Autodesk Inventor part; units mm, degrees
ref_plane "Work Plane1" through (119.25, -2.5, 0) normal (1, 0, 0) x (0, 0, -1)
ref_plane "YZ Plane" through (0, 0, 0) normal (1, 0, 0) x (0, 1, 0)
ref_plane "XZ Plane" through (0, 0, 0) normal (0, 1, 0) x (-1, 0, 0)
sketch "Sketch2" plane through (0, 0, 0) normal (0, 0, 1) x (1, 0, 0)
  line L0 (-124.5, 2.5) -> (124.5, 2.5)
  line L1 (124.5, 2.5) -> (124.5, -2.5)
  line L2 (124.5, -2.5) -> (-124.5, -2.5)
  line L3 (-124.5, -2.5) -> (-124.5, 2.5)
  point P0 (0, 0)
  dimension "d1" = 249
  dimension "d2" = 5
  dimension "d3" = 2.5
  dimension "d4" = 124.5
sketch "Sketch3" plane through (0, 0, 0) normal (1, 0, 0) x (0, 1, 0)
  line L0 (0, 0) -> (-53.033, 53.033)
  line L1 (0, -0.5221) -> (1.6531, -0.5221)
  dimension "d5" = 75
  dimension "d6" = 45
sweep "Sweep1" add profiles "Sketch2" path "Sketch3" path curves L0
sketch "Sketch10" plane through (124.5, 2.5, 0) normal (0, 0, -1) x (-1, 0, 0)
  line L0 (249, 0) -> (0, 0)
  line L1 (0, 0) -> (0, -5)
  line L2 (0, -5) -> (249, -5)
  line L3 (249, -5) -> (249, 0)
  line L4 (15, 0) -> (234, 0)
  line L5 (234, 0) -> (234, -2)
  line L6 (234, -2) -> (15, -2)
  line L7 (15, -2) -> (15, 0)
  point P0 (124.5, -2.5)
  dimension "d76" = 2
  dimension "d77" = 219
  dimension "d78" = 109.5
extrude "Extrusion5" add sketch "Sketch10" along normal blind 10 contours L5 L6 L7 L0
sketch "Sketch11" plane through (-109.5, 0.5, 0) normal (0, -1, 0) x (1, 0, 0)
  line L0 (0, 0) -> (219, 0)
  line L1 (0, 0) -> (0, -10)
  line L2 (219, -10) -> (0, -10)
  line L3 (219, 0) -> (219, -10)
  line L4 (201.75, -6) -> (151.75, -6)
  line L5 (151.75, -6) -> (151.75, -4)
  line L6 (151.75, -4) -> (201.75, -4)
  line L7 (201.75, -4) -> (201.75, -6)
  line L8 (134.5, -6) -> (84.5, -6)
  line L9 (84.5, -6) -> (84.5, -4)
  line L10 (84.5, -4) -> (134.5, -4)
  line L11 (134.5, -4) -> (134.5, -6)
  line L12 (67.25, -6) -> (17.25, -6)
  line L13 (17.25, -6) -> (17.25, -4)
  line L14 (17.25, -4) -> (67.25, -4)
  line L15 (67.25, -4) -> (67.25, -6)
  point P0 (109.5, 0)
  dimension "d81" = 50
  dimension "d82" = 2
  dimension "d83" = 10
  dimension "d84" = 219
  dimension "d85" = 4
  dimension "d86" = 50
  dimension "d87" = 50
  dimension "d88" = 17.25
  dimension "d89" = 17.25
  dimension "d90" = 17.25
  dimension "d91" = 17.25
extrude "Extrusion6" add sketch "Sketch11" along normal blind 6 contours L4 L5 L6 L7 | L8 L9 L10 L11 | L12 L13 L14 L15
sketch "Sketch13" plane through (124.5, -2.5, 0) normal (1, 0, 0) x (0, 0, -1)
  line L0 (0, 5) -> (0, 0)
  line L1 (0, 5) -> (-53.033, -48.033)
  line L2 (-53.033, -53.033) -> (-53.033, -48.033)
  line L3 (0, 0) -> (-53.033, -53.033)
  line L4 (-7.0711, -2.0711) -> (-7.0711, -4.5711)
  line L5 (-7.0711, -4.5711) -> (-45.9619, -43.4619)
  line L6 (-45.9619, -43.4619) -> (-45.9619, -40.9619)
  line L7 (-7.0711, -3.3211) -> (0, 3.75)
  line L8 (-45.9619, -42.2119) -> (-53.033, -49.283)
  point P0 (0, 2.5)
  dimension "d98" = 2.5
  dimension "d99" = 10
  dimension "d101" = 2.5
  dimension "d102" = 10
  dimension "d103" = 45
extrude "Extrusion7" cut sketch "Sketch13" against normal blind 10.5 contours L4 L5 L6 L1
ref_plane "Work Plane1" through (119.25, -2.5, 0) normal (1, 0, 0) x (0, 0, -1)
sketch "Sketch14" plane through (119.25, -2.5, 0) normal (1, 0, 0) x (0, 0, -1)
  line L0 (-7.0711, -2.0711) -> (-7.0711, -4.5711)
  line L1 (-7.0711, -4.5711) -> (-45.9619, -43.4619)
  line L2 (-45.9619, -43.4619) -> (-45.9619, -40.9619)
  line L3 (-45.9619, -40.9619) -> (-53.033, -48.033)
  line L4 (-53.033, -53.033) -> (-53.033, -48.033)
  line L5 (0, 0) -> (-53.033, -53.033)
  line L6 (0, 5) -> (0, 0)
  line L7 (0, 5) -> (-7.0711, -2.0711)
  line L8 (-45.9619, -40.9619) -> (-7.0711, -2.0711)
  line L9 (-45.9619, -43.4619) -> (-45.9619, -40.9619)
  line L10 (-7.0711, -4.5711) -> (-45.9619, -43.4619)
  line L11 (-7.0711, -2.0711) -> (-7.0711, -4.5711)
  line L12 (-13.0815, -10.5815) -> (-13.0815, -13.0815)
  line L13 (-23.6881, -21.1881) -> (-23.6881, -23.6881)
  line L14 (-29.3449, -26.8449) -> (-29.3449, -29.3449)
  line L15 (-39.9515, -37.4515) -> (-39.9515, -39.9515)
  line L16 (-23.6881, -21.1881) -> (-13.0815, -10.5815)
  line L17 (-13.0815, -13.0815) -> (-23.6881, -23.6881)
  line L18 (-29.3449, -26.8449) -> (-39.9515, -37.4515)
  line L19 (-29.3449, -29.3449) -> (-39.9515, -39.9515)
  line L20 (-39.9515, -39.9515) -> (-39.9515, -37.4515)
  line L21 (-39.9515, -37.4515) -> (-29.3449, -26.8449)
  line L22 (-29.3449, -26.8449) -> (-29.3449, -29.3449)
  line L23 (-29.3449, -29.3449) -> (-39.9515, -39.9515)
  line L24 (-23.6881, -21.1881) -> (-13.0815, -10.5815)
  line L25 (-13.0815, -10.5815) -> (-13.0815, -13.0815)
  line L26 (-13.0815, -13.0815) -> (-23.6881, -23.6881)
  line L27 (-23.6881, -23.6881) -> (-23.6881, -21.1881)
  point P0 (0, 2.5)
  dimension "d106" = 15
  dimension "d107" = 15
  dimension "d109" = 55
  dimension "d110" = 8.5
  dimension "d111" = 8.5
  dimension "d112" = 8
extrude "Extrusion8" cut sketch "Sketch14" along normal mid plane 3 contours L12 L5 L13 L1 | L1 L14 L5 L15
mirror "Mirror2" about plane through (0, 0, 0) normal (1, 0, 0) of "Extrusion8", "Extrusion7"
ref_plane "Work Plane2" through (-119.25, -2.5, 0) normal (1, 0, 0) x (0, 0, -1)
equation "\"d85\" = -0.5 * d82 + 0.5 * d83"
equation "\"d86\" = d81"
equation "\"d87\" = d81"
equation "\"d88\" = -0.75 * d81 + 0.25 * d84"
equation "\"d89\" = d88"
equation "\"d90\" = d88"
equation "\"d111\" = d110"
properties part number "Roof Length Extension"
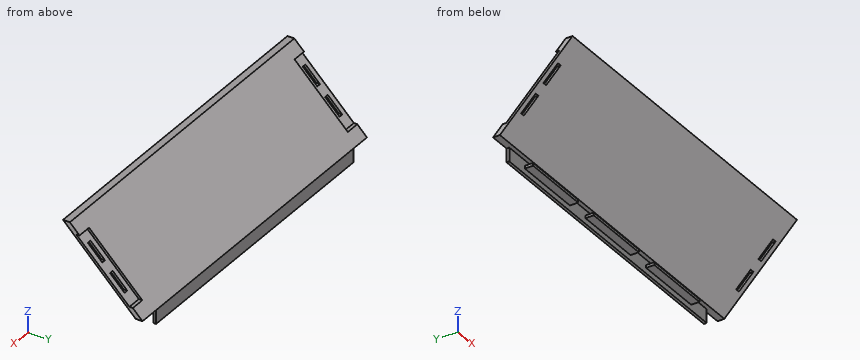
The listing builds one solid part. Answer for the finished solid, in the listing's coordinates (mm). Give positions to 0.01 mm unless a question says otherwise; leave off trailing zeros. Order: outer loops, then holes, each group sorted by start corner. A loop starts at its lowest first (then second) coordinate and runs counter-clockwise, first axis right, second up. Notation, with made-up numbers: M -10,21 L 47,21 A31 cw 47,49 Z; hole C -1.5,71.25 d9. An arc over 180 degrees is marked long. Put each result on its own line as item: value. Start each with the question number.
Item 1: Flat-ended cylindrical pins translate along their axes: P1, Ø3, axis at x = -21, y = -34.5, coming from the +Z side; P2, Ø1, axis at y = 1, z = -3, coming from the +X side; P3, Ø1.5, axis at x = 85.5, z = 20.5, coming from the -Y side. Find the tip coordinate at first contact, or state that the pin passes through.
Item 2: The part is cut by section B-B, the plane x = -107. Determine the outline of the cut face in (y, z).
Item 3: The part is cut by section A-A, the plane z = 32.5. Determine the outline of the cut face in (x, y).
Item 4: The part is cut by section D-D, the plane z = 42.5. Determine the outline of the cut face in (x, y).
Item 5: Find the intervals of material crossed by line 1 along Y through (x, z) = (-42, -2.5); line 2 along Y through (x, z) = (27.5, 13.5); line 3 along Z through (x, y) = (-48, -23), in increasing order.
Item 6: The part is cut by section C-C, the plane y = -10. Determine the outline of the cut face in (x, z), and give its area (3 significant figures).
Answer key:
1. P1: stops at z = 38.5
1. P2: stops at x = 109.5
1. P3: stops at y = -23.75
2. outline: M -55.53,53.03 L -2.5,0 L 0.5,0 L 0.5,-10 L 2.5,-10 L 2.5,0 L -50.53,53.03 Z
3. outline: M -124.5,-35 L -120.75,-35 L -120.75,-32.5 L -124.5,-32.5 Z; M -117.75,-35 L 117.75,-35 L 117.75,-32.5 L 114,-32.5 L 114,-30 L -114,-30 L -114,-32.5 L -117.75,-32.5 Z; M 120.75,-35 L 124.5,-35 L 124.5,-32.5 L 120.75,-32.5 Z
4. outline: M -124.5,-45 L 124.5,-45 L 124.5,-42.5 L 114,-42.5 L 114,-40 L -114,-40 L -114,-42.5 L -124.5,-42.5 Z
5. line 1: y = 0.5 to 2.5
5. line 2: y = -16 to -11
5. line 3: z = 20.5 to 25.5
6. outline: M -124.5,7.5 L 124.5,7.5 L 124.5,10 L 114,10 L 114,12.5 L -114,12.5 L -114,10 L -124.5,10 Z
6. area: 1,190 mm²
